Can you work these out from the model? Positions are in its coordinate system, mm. A direction names the side the tool comes from. Round coordinates to 2 decimals unless told otherwise and drop trailing zeros. Write each loop counter-clockwise with the first axis right and the second up, starting at its lowest first coordinate (ties: lowest second). Pieces come first, ordered by that corner, then holes. Notation, with made-up numbers: M -30.5,-32 L 14.5,-32 A36 ccw 14.5,5 Z; hole C -23,72 d8. An arc over 180 degrees is marked long. Use one line per item in the form item = value. Start each with the question number.
```python
from build123d import *

# Parameters (mm, degrees)
BOSS_EXTRUDE1_DEPTH = 52
CUT_EXTRUDE1_REACH  = 67.031
SKETCH2_R           = 1.8
CUT_EXTRUDE3_REACH  = 67.031
SKETCH4_R           = 1.35
CUT_EXTRUDE4_REACH  = 67.031
SKETCH5_R           = 1.35
SKETCH6_R           = 1.35
CUT_EXTRUDE5_DEPTH  = 64.277168192
CHAMFER3_SIZE       = 12
LPATTERN3_COUNT     = 2
LPATTERN3_PITCH     = 22
LPATTERN3_COL_COUNT = 2
LPATTERN3_COL_PITCH = 22
SKETCH7_W           = 5.8
SKETCH7_H           = 12
SKETCH7_H_2         = 12.747013555
SKETCH7_H_3         = 13.058470869
CUT_EXTRUDE6_DEPTH  = 2.5
CHAMFER4_SIZE       = 2.5


# Some blends are built 0.0001 mm under size
with BuildPart() as part:
    # Sketch1 → Boss-Extrude1 (new body)
    with BuildSketch(Plane.XY):
        with BuildLine():
            Line((0, 0), (25, 0))
            ThreePointArc((25, 0), (28.535533906, 1.464466094), (30, 5))
            Line((30, 5), (30, 11))
            ThreePointArc((30, 11), (28.535533906, 14.535533906), (25, 16))
            Line((25, 16), (8, 16))
            ThreePointArc((8, 16), (6, 18), (8, 20))
            Line((8, 20), (20, 20))
            Line((20, 20), (20, 25))
            Line((20, 25), (0, 25))
            Line((0, 25), (0, 17.6))
            ThreePointArc((0, 17.6), (1.171572875, 14.771572875), (4, 13.6))
            Line((4, 13.6), (20, 13.6))
            ThreePointArc((20, 13.6), (24.3, 9.3), (20, 5))
            Line((20, 5), (0, 5))
            Line((0, 5), (0, 0))
        make_face()
    extrude(amount=BOSS_EXTRUDE1_DEPTH)

    # Cut-Extrude1: up to this face of the body (flat: up to its plane)
    cut_extrude1_end = Plane(part.part.faces().sort_by_distance((12, 13.6, 26))[0])
    # Sketch2 → Cut-Extrude1 (cut, up to the picked face)
    with BuildSketch(Plane(origin=(0, 25, 0), x_dir=(1, 0, 0), z_dir=(0, 1, 0)), mode=Mode.PRIVATE) as cut_extrude1_sk1:
        with Locations(Location((16, -26, 0), (0, 0, 270))):
            Circle(SKETCH2_R)
    cut_extrude1_tool1 = split(extrude(cut_extrude1_sk1.sketch, amount=-CUT_EXTRUDE1_REACH, mode=Mode.PRIVATE), bisect_by=cut_extrude1_end, keep=Keep.BOTH, mode=Mode.PRIVATE)
    cut_extrude1 = cut_extrude1_tool1.solids().sort_by(Axis((16, 25, 26), (0, -1, 0)))[0]
    add(cut_extrude1, mode=Mode.SUBTRACT)

    # Sketch4 → Cut-Extrude3 (cut, up to next)
    with BuildSketch(Plane(origin=(0, 25, 0), x_dir=(1, 0, 0), z_dir=(0, 1, 0)), mode=Mode.PRIVATE) as cut_extrude3_sk1:
        with Locations(Location((3, -26, 0), (0, 0, 270))):
            Circle(SKETCH4_R)
    cut_extrude3_tool1 = extrude(cut_extrude3_sk1.sketch, amount=-CUT_EXTRUDE3_REACH, mode=Mode.PRIVATE) & part.part
    cut_extrude3 = cut_extrude3_tool1.solids().sort_by_distance((3, 25, 26))[0]
    add(cut_extrude3, mode=Mode.SUBTRACT)

    # Sketch5 → Cut-Extrude4 (cut, up to next)
    with BuildSketch(Plane.XZ, mode=Mode.PRIVATE) as cut_extrude4_sk1:
        with Locations(Location((3, 26, 0), (0, 0, 90))):
            Circle(SKETCH5_R)
    cut_extrude4_tool1 = extrude(cut_extrude4_sk1.sketch, amount=-CUT_EXTRUDE4_REACH, mode=Mode.PRIVATE) & part.part
    cut_extrude4 = cut_extrude4_tool1.solids().sort_by_distance((3, 0, 26))[0]
    add(cut_extrude4, mode=Mode.SUBTRACT)

    # Sketch6 → Cut-Extrude5 (cut, through all)
    with BuildSketch(Plane(origin=(0, 5, 0), x_dir=(1, 0, 0), z_dir=(0, 1, 0))):
        with Locations(Location((16, -26, 0), (0, 0, 180))):
            Circle(SKETCH6_R)
    cut_extrude5 = extrude(amount=-CUT_EXTRUDE5_DEPTH, mode=Mode.SUBTRACT)

    # Chamfer3
    # the kernel refuses this chamfer: 12 mm, written as the material it takes off along each edge
    with BuildSketch(Plane(origin=(30, -25.860195856, 0), x_dir=(-0.9996219169112969, 0, -0.027495876610586372), z_dir=(0, 1, 0))) as chamfer3_piece_1_section:
        Polygon((CHAMFER3_SIZE * 0.999621916911, CHAMFER3_SIZE * 0.0274958766106), (-CHAMFER3_SIZE * 0.0274958766106, CHAMFER3_SIZE * 0.999621916911), (0, 0), align=None)
    chamfer3_piece_1 = extrude(amount=67.720391711, mode=Mode.PRIVATE)
    chamfer3_piece_1 = split(chamfer3_piece_1, bisect_by=Plane(origin=(19.333333334, 20, 0.666666666), z_dir=(0, -1, 0)), keep=Keep.TOP, mode=Mode.PRIVATE)
    add(chamfer3_piece_1, mode=Mode.SUBTRACT)
    with BuildSketch(Plane(origin=(30, -25.860195856, 52), x_dir=(-0.9996219169112969, 0, 0.027495876610586202), z_dir=(0, 1, 0))) as chamfer3_piece_2_section:
        Polygon((CHAMFER3_SIZE * 0.999621916911, -CHAMFER3_SIZE * 0.0274958766106), (-CHAMFER3_SIZE * 0.0274958766106, -CHAMFER3_SIZE * 0.999621916911), (0, 0), align=None)
    chamfer3_piece_2 = extrude(amount=67.720391711, mode=Mode.PRIVATE)
    chamfer3_piece_2 = split(chamfer3_piece_2, bisect_by=Plane(origin=(19.333333334, 20, 51.333333333), z_dir=(0, -1, 0)), keep=Keep.TOP, mode=Mode.PRIVATE)
    add(chamfer3_piece_2, mode=Mode.SUBTRACT)

    # LPattern3: Cut-Extrude1, Cut-Extrude3, Cut-Extrude4, Cut-Extrude5 ×2
    with Locations(*[(0, 0, i * LPATTERN3_PITCH) for i in range(1, LPATTERN3_COUNT)]):
        add(cut_extrude1, mode=Mode.SUBTRACT)
        add(cut_extrude3, mode=Mode.SUBTRACT)
        add(cut_extrude4, mode=Mode.SUBTRACT)
        add(cut_extrude5, mode=Mode.SUBTRACT)

    # LPattern3 col: Cut-Extrude1, Cut-Extrude3, Cut-Extrude4, Cut-Extrude5 ×2
    with Locations(*[(0, 0, -i * LPATTERN3_COL_PITCH) for i in range(1, LPATTERN3_COL_COUNT)]):
        add(cut_extrude1, mode=Mode.SUBTRACT)
        add(cut_extrude3, mode=Mode.SUBTRACT)
        add(cut_extrude4, mode=Mode.SUBTRACT)
        add(cut_extrude5, mode=Mode.SUBTRACT)

    # Sketch7 → Cut-Extrude6 (cut)
    with BuildSketch(Plane.XZ):
        with Locations((16, 26)):
            Rectangle(SKETCH7_W, SKETCH7_H)
        with Locations((16, 4.626493222)):
            Rectangle(SKETCH7_W, SKETCH7_H_2)
        with Locations((16, 47.529235435)):
            Rectangle(SKETCH7_W, SKETCH7_H_3)
    extrude(amount=-CUT_EXTRUDE6_DEPTH, mode=Mode.SUBTRACT)

    # Chamfer4
    chamfer4_edges = [part.edges().sort_by_distance(p)[0] for p in [
        (16, 2.5, 41),
        (16, 2.5, 20),
        (16, 2.5, 32),
        (16, 2.5, 11),
    ]]
    chamfer(chamfer4_edges, length=CHAMFER4_SIZE - 0.0001)  # a hair under: the kernel refuses the full size


solid = part.part
```
1. Please list where these lines run through material, in increasing order: line 1 along Z through (x, y) = (3, 18.25); line 2 along Y through (x, z) = (11, 40.5); line 3 along Y through (x, z) = (13.5, 46.5).
2. If we section it at A-A (x = 9.5): List the corners of the cut face in (y, z) for me, and give its area (3 significant figures).
3. If we mould it in two halves opening along X, with no side actions, what happens to faces 1 (the face through (14.7, 2.5, 5.3)), 2 (the face through (18.9, 1, 47)), 3 (the face through (29, 14, 26)), 4 (the face through (1.141, 14.803, 25.636))? For each: pulls with the +X half, pulls with the -X half, needs draft (parallel to the pull), parting line crosses it, or undercut.
4. If we section it at D-D (x = 16): State how many separate pieces and enclosed holes the cut face has, and give its area (3 significant figures).
5. If we section it at B-B (y = 18.25): List the corners of the cut face in (x, z) for me.
6. If we section it at C-C (z = 33): List the corners of the cut face in (x, y) for me, and give its area (3 significant figures).
7. Which directions (+Z, -Z, +X, -X, +Y, -Y) give clear straight access to the entire face, cutting with the end or side of a thin tool? Please do faces 5 (the face through (18.9, 1, 26)), 6 (the face through (25, 8, 45)), 7 (the face through (19, 16, 26)), 8 (the face through (16, 1, 42)).
8. Will these pins go through, and if not, where does the flat tip stop? pin 1 (3.5 mm diameter, centred on x = 16, z = 26, fed in from +Y); pin 2 (3 mm diameter, centred on x = 16, z = 4, fed in from -Y); pin 3 (1.6 mm diameter, centred on x = 16, z = 48, fed in from -Y); pin 4 (2 mm diameter, centred on y = 1, z = 28.5, fed in from +X).
Model answer:
q1.line_1 = 0 to 2.65, 5.35 to 24.65, 27.35 to 46.65, 49.35 to 52
q1.line_2 = 0 to 5, 13.6 to 16, 20 to 25
q1.line_3 = 2.5 to 5, 13.6 to 16, 20 to 25
q2.outline = M 0,0 L 5,0 L 5,52 L 0,52 Z; M 13.6,0 L 16,0 L 16,52 L 13.6,52 Z; M 20,0 L 25,0 L 25,52 L 20,52 Z
q2.area = 645 mm2
q3.face_1 = undercut
q3.face_2 = undercut
q3.face_3 = pulls with the +X half
q3.face_4 = pulls with the -X half
q4.separate_pieces = 12
q4.enclosed_holes = 0
q4.area = 472 mm2
q5.outline = M 0,0 L 6.02,0 L 6.02,52 L 0,52 Z; hole C 3,4 d2.7; hole C 3,26 d2.7; hole C 3,48 d2.7
q6.outline = M 0,0 L 25,0 A5 ccw 30,5 L 30,11 A5 ccw 25,16 L 8,16 A2 cw 8,20 L 20,20 L 20,25 L 0,25 L 0,17.6 A4 ccw 4,13.6 L 20,13.6 A4.3 cw 20,5 L 0,5 Z
q6.area = 391 mm2
q7.face_5 = -Y
q7.face_6 = +Z, +X, -Y
q7.face_7 = +Z, -Z, +X
q7.face_8 = +Z, -Y
q8.pin_1 = 5
q8.pin_2 = 2.5
q8.pin_3 = through
q8.pin_4 = 29
